from build123d import *

# Parameters (mm, degrees)
SKETCH_W        = 42
SKETCH_H        = 52
SKETCH_R        = 1.75
PAD_DEPTH       = 7
SKETCH001_R     = 3.25
POCKET_DEPTH    = 3
POCKET001_DEPTH = 7.001
FILLET_R        = 5
FILLET001_R     = 2
CHAMFER_SIZE    = 0.5
CHAMFER001_SIZE = 0.5
CHAMFER002_SIZE = 0.5
CHAMFER003_SIZE = 0.5
SKETCH003_R     = 1.75
PAD001_DEPTH    = 0.3


with BuildPart() as part:
    # Sketch → Pad (new body)
    with BuildSketch(Plane.XY):
        with Locations((0, -5)):
            Rectangle(SKETCH_W, SKETCH_H)
        with Locations((-15.5, 15.5)):
            Circle(SKETCH_R, mode=Mode.SUBTRACT)
        with Locations((15.5, 15.5)):
            Circle(SKETCH_R, mode=Mode.SUBTRACT)
        with Locations((15.5, -15.5)):
            Circle(SKETCH_R, mode=Mode.SUBTRACT)
        with Locations((-15.5, -15.5)):
            Circle(SKETCH_R, mode=Mode.SUBTRACT)
        with Locations((-15.5, -26)):
            Circle(SKETCH_R, mode=Mode.SUBTRACT)
        with Locations((15.5, -26)):
            Circle(SKETCH_R, mode=Mode.SUBTRACT)
    extrude(amount=PAD_DEPTH)

    # Sketch001 → Pocket (cut)
    with BuildSketch(Plane(origin=(0, 0, 0), x_dir=(1, 0, 0), z_dir=(0, 0, -1))):
        with Locations((-15.5, 15.5)):
            Circle(SKETCH001_R)
        with Locations((15.5, 15.5)):
            Circle(SKETCH001_R)
    extrude(amount=-POCKET_DEPTH, mode=Mode.SUBTRACT)

    # Sketch002 → Pocket001 (cut, through all)
    with BuildSketch(Plane.XY.offset(7)):
        with BuildLine():
            ThreePointArc((-6, -21), (-9.5, -24.5), (-6, -28))
            Line((-6, -28), (6, -28))
            ThreePointArc((6, -28), (9.5, -24.5), (6, -21))
            Line((-6, -21), (6, -21))
        make_face()
        with BuildLine():
            ThreePointArc((-16.5, 10.091673), (-11.610913, 11.610913), (-10.091673, 16.5))
            Line((10.091673, 16.5), (-10.091673, 16.5))
            ThreePointArc((10.091673, 16.5), (11.610913, 11.610913), (16.5, 10.091673))
            Line((16.5, -10.091673), (16.5, 10.091673))
            ThreePointArc((16.5, -10.091673), (11.610913, -11.610913), (10.091673, -16.5))
            Line((-10.091673, -16.5), (10.091673, -16.5))
            ThreePointArc((-10.091673, -16.5), (-11.610913, -11.610913), (-16.5, -10.091673))
            Line((-16.5, 10.091673), (-16.5, -10.091673))
        make_face()
    extrude(amount=-POCKET001_DEPTH, mode=Mode.SUBTRACT)

    # Fillet
    fillet_edges = [part.edges().sort_by_distance(p)[0] for p in [
        (-21, -31, 3.5),
        (21, -31, 3.5),
        (21, 21, 3.5),
        (-21, 21, 3.5),
    ]]
    fillet(fillet_edges, radius=FILLET_R)

    # Fillet001
    fillet001_edges = [part.edges().sort_by_distance(p)[0] for p in [
        (-10.091673, -16.5, 3.5),
        (-16.5, -10.091673, 3.5),
        (-16.5, 10.091673, 3.5),
        (-10.091673, 16.5, 3.5),
        (10.091673, 16.5, 3.5),
        (16.5, 10.091673, 3.5),
        (16.5, -10.091673, 3.5),
        (10.091673, -16.5, 3.5),
    ]]
    fillet(fillet001_edges, radius=FILLET001_R)

    # Chamfer
    chamfer_edges = [part.edges().sort_by_distance(p)[0] for p in [
        (21, -5, 0),
    ]]
    chamfer(chamfer_edges, length=CHAMFER_SIZE)

    # Chamfer001
    chamfer001_edges = [part.edges().sort_by_distance(p)[0] for p in [
        (-16.5, 0, 0),
    ]]
    chamfer(chamfer001_edges, length=CHAMFER001_SIZE)

    # Chamfer002
    chamfer002_edges = [part.edges().sort_by_distance(p)[0] for p in [
        (-18.75, -15.5, 0),
        (12.25, -15.5, 0),
        (-17.25, 15.5, 0),
        (13.75, 15.5, 0),
        (13.75, -26, 0),
        (-17.25, -26, 0),
    ]]
    chamfer(chamfer002_edges, length=CHAMFER002_SIZE)

    # Chamfer003
    chamfer003_edges = [part.edges().sort_by_distance(p)[0] for p in [
        (0, -21, 0),
    ]]
    chamfer(chamfer003_edges, length=CHAMFER003_SIZE)

    # Sketch003 → Pad001 (new body)
    with BuildSketch(Plane(origin=(0, 0, 3), x_dir=(1, 0, 0), z_dir=(0, 0, -1))):
        with Locations((-15.5, 15.5)):
            Circle(SKETCH003_R)
        with Locations((15.5, 15.5)):
            Circle(SKETCH003_R)
    extrude(amount=-PAD001_DEPTH)


solid = part.part
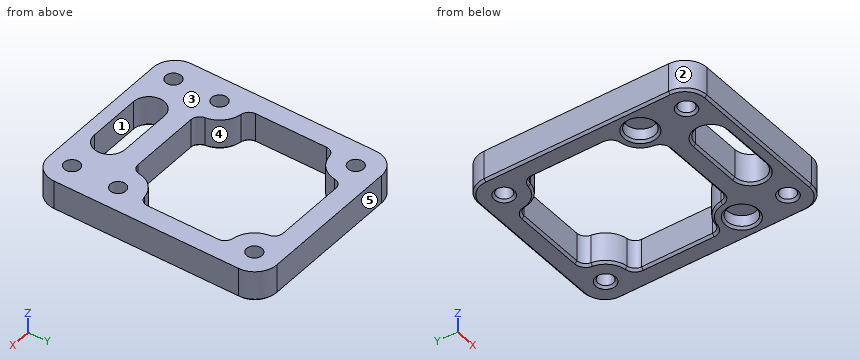
For this review, take the finished solid that the model builds, in its own axes (mm). Face numbers are marked on the shaded views. A direction names the side the tool comes from. Coordinates: 2 decimals unless noted, no trailing zeros. Write each loop counter-clockwise with the first axis right and the second up, starting at its lowest first coordinate (ties: lowest second). Pieces come first, ordered by that corner, then holes. Notation, with made-up numbers: (86, -12.5) -> (129, -12.5) arc R31 cw to (129, 14.5) -> close; hole circle Ø1 at (21.25, 48.25). An arc over 180 degrees is marked (long way). Write each question's results on one line, items separated by ' | '. Start each with the question number.
1) Consider section C-C (x = 0.5). Write out the cut boundary in (y, z).
2) Consider section A-A (y = -1.5). Write out the cut boundary in (x, z), plus the area to 3 significant figures.
3) Consider section B-B (z = 2). Give the number of separate pieces and of enclosed holes in the cut face, plus the area to 3 significant figures.
4) Insertion check: pin 1 (5.5 mm diameter, centred on x = -15.5, y = -15.5, fed in from -Z); pin 2 (7.5 mm diameter, centred on x = -15.5, y = -15.5, fed in from +Z); pin 3 (1 mm diameter, centred on x = 16, y = -16, fed in from +Z). Each pin has a flat end and moves straight along its axis. Give the tip position at first contact, or say it passes through.
5) Wall thickness on L1, parallel to Y at x = 5.5, z = 2; L2, parallel to X at y = 3, z = 3; L3, parallel to Y at x = -15.5, z = 2: over which ranges is each line inside the solid? List them lowest first. Write a range as [from, to].
6) For the marked faces 4 and 5, list the 3-axis set-ups (+Z, -Z, +X, -X, +Y, -Y) from which the entire face can be reached by the end or side of a thin tool; tool diameter is ignored.
7) The part is to be moulded in two halves that separate along Y. For the marked faces 1, 2 and 3, say which applies: +Y half, -Y half, draft (parallel to the pull), parting line (faces both ways), or undercut.
Geometry says:
1) outline: (-31, 0.5) -> (-30.5, 0) -> (-28.5, 0) -> (-28, 0.5) -> (-28, 7) -> (-31, 7) -> close; (-21, 0.5) -> (-20.5, 0) -> (-17, 0) -> (-16.5, 0.5) -> (-16.5, 7) -> (-21, 7) -> close; (16.5, 0.5) -> (17, 0) -> (20.5, 0) -> (21, 0.5) -> (21, 7) -> (16.5, 7) -> close
2) outline: (-21, 0.5) -> (-20.5, 0) -> (-17, 0) -> (-16.5, 0.5) -> (-16.5, 7) -> (-21, 7) -> close; (16.5, 0.5) -> (17, 0) -> (20.5, 0) -> (21, 0.5) -> (21, 7) -> (16.5, 7) -> close | area: 62.5 mm^2
3) separate pieces: 1 | enclosed holes: 8 | area: 995 mm^2
4) pin 1: z = 3 | pin 2: z = 7 | pin 3: z = 3.3
5) L1: [-31, -28], [-21, -16.5], [16.5, 21] | L2: [-21, -16.5], [16.5, 21] | L3: [-31, -27.75], [-24.25, -18.75], [-12.25, -9.8], [9.8, 13.75], [17.25, 21]
6) face 4: +Z, -Z | face 5: +Z, -Z, +X, -X, +Y
7) face 1: undercut | face 2: -Y half | face 3: draft
